```python
from build123d import *

# Parameters (mm, degrees)
SKETCH1_R           = 2.8
SKETCH1_R_2         = 1.5
BOSS_EXTRUDE3_DEPTH = 4
BOSS_EXTRUDE5_DEPTH = 10


with BuildPart() as part:
    # Sketch1 → Boss-Extrude3 (new body)
    with BuildSketch(Plane.XY):
        with BuildLine():
            Line((-5.977999231, 22.118015055), (-5.977999231, 19.918015055))
            ThreePointArc((-5.977999231, 19.918015055), (0.022000769, 13.918015055), (6.022000769, 19.918015055))
            Line((6.022000769, 19.918015055), (6.022000769, 22.118015055))
            ThreePointArc((6.022000769, 22.118015055), (0.022000769, 28.118015055), (-5.977999231, 22.118015055))
        make_face()
        with Locations((0.022000769, 19.918015055)):
            Circle(SKETCH1_R, mode=Mode.SUBTRACT)
        with Locations((0.022000769, 25.418015055)):
            Circle(SKETCH1_R_2, mode=Mode.SUBTRACT)
    extrude(amount=BOSS_EXTRUDE3_DEPTH)

    # Sketch1<8> → Boss-Extrude5 (add)
    with BuildSketch(Plane.XY):
        with BuildLine():
            ThreePointArc((-2.374426324, 22.867105964), (0.022000769, 16.118015055), (2.418427861, 22.867105964))
            ThreePointArc((2.418427861, 22.867105964), (2.004907724, 22.533906873), (1.545736934, 22.267105964))
            ThreePointArc((1.545736934, 22.267105964), (0.022000769, 17.118015055), (-1.501735396, 22.267105964))
            ThreePointArc((-1.501735396, 22.267105964), (-1.960906186, 22.533906873), (-2.374426324, 22.867105964))
        make_face()
    extrude(amount=BOSS_EXTRUDE5_DEPTH)


solid = part.part
```
Input: part model. Units: mm. Frame: model coordinates. A direction names the side the tool comes from. Give positions to 0.01 mm unless a question says otherwise; leave off trailing zeros. Write each loop counter-clockwise with the first axis right and the second up, starting at its lowest first coordinate (ties: lowest second). Pieces come first, ordered by that corner, then holes. Notation, with made-up numbers: (42.25, 7) - (69.25, 7) arc R27 ccw to (69.25, 40) - close; hole circle Ø8 at (59, -11). An arc over 180 degrees is marked (long way). Write item = value, one per line. Start each with the question number.
1. Section query B-B, the plane x = -3.25. Output: boundary loops of the cut face in (y, z), then the cut area to 3 significant figures.
2. Ray query, L1, parallel to X at y = 20, z = 2.5; L2, parallel to Y at x = -0.5, z = 0.75; L3, parallel to Y at x = -1, z = 1.5. Return the intervals inside material, ascending.
3. Access query for faces 1 (the flat face through (-5.978, 21, 2)), 2 (the cylindrical face through (-1.955, 22.53, 6.958)), 3 (the cylindrical face through (-0.11, 16.12, 6.96)). Directions: +Z, -Z, +X, -X, +Y, -Y. A direction counts if a zero-diameter tool reaches every point of the face in a straight line with its end or side. Return the directions, or none.
4. First-contact query: pin 1 Ø5 at (y, z) = (26.5, 4) entering from +X; pin 2 Ø6 at (x, z) = (4.5, 2) entering from -Y. Flat tips, straight axial feed; report the tip coordinate or a pass-through.
5. Mould query, pull axis Y, two halves, no side actions, for faces 4 (the cylindrical face through (-0.11, 13.92, 1.97)), 5 (the cylindrical face through (2.011, 22.538, 6.958)), 6 (the cylindrical face through (2.72, 19.17, 4.93)), 7 (the cylindrical face through (-0.303, 23.954, 1.972)). Classes: released by +Y, released by -Y, zero draft, split by the parting line, or undercut.
6. Section query C-C, the plane y = 21.25. Output: boundary loops of the cut face in (x, z), then the cut area to 3 significant figures.
7. Section query A-A, the plane y = 26. Output: boundary loops of the cut face in (x, z).
8. Section query D-D, the plane z = 1. Output: boundary loops of the cut face in (x, y).
Check sheet entries:
q1.outline = (14.89, 0) - (27.15, 0) - (27.15, 4) - (21.85, 4) - (21.85, 10) - (17.99, 10) - (17.99, 4) - (14.89, 4) - close
q1.area = 72.2 mm2
q2.L1 = -5.98 to -2.78, 2.82 to 6.02
q2.L2 = 13.94 to 17.17, 22.67 to 24.01, 26.82 to 28.1
q2.L3 = 14.01 to 17.31, 22.52 to 24.32, 26.52 to 28.03
q3.face_1 = +Z, -Z, -X, +Y, -Y
q3.face_2 = +Z, +Y
q3.face_3 = +Z
q4.pin_1 = 5.72
q4.pin_2 = 14.1
q5.face_4 = released by -Y
q5.face_5 = released by +Y
q5.face_6 = undercut
q5.face_7 = undercut
q6.outline = (-5.98, 0) - (-2.44, 0) - (-2.44, 10) - (-3.54, 10) - (-3.54, 4) - (-5.98, 4) - close; (2.48, 0) - (6.02, 0) - (6.02, 4) - (3.58, 4) - (3.58, 10) - (2.48, 10) - close
q6.area = 41.4 mm2
q7.outline = (-4.55, 0) - (-1.36, 0) - (-1.36, 4) - (-4.55, 4) - close; (1.4, 0) - (4.6, 0) - (4.6, 4) - (1.4, 4) - close
q8.outline = (-5.98, 19.92) arc R6 ccw to (6.02, 19.92) - (6.02, 22.12) arc R6 ccw to (-5.98, 22.12) - close; hole circle Ø5.6 at (0.02, 19.92); hole circle Ø3 at (0.02, 25.42)
